The listing builds one solid part. Answer for the finished solid, in the listing's coordinates (mm). A direction names the side the tool comes from. Coordinates: 2 decimals unless noted, no trailing zeros. Order: outer loops, then holes, each group sorted by start corner. A loop starts at its lowest first (then second) coordinate and runs counter-clockwise, first axis right, second up. Notation, with made-up numbers: (-8.5, 15) -> (15.5, 15) arc R23 cw to (15.5, 23) -> close; hole circle Ø3 at (70, -28). An arc over 180 degrees is marked (long way). Return JSON: item names as keys, results as strings.
```python
from build123d import *

# Parameters (mm, degrees)
SKETCH2_R               = 6.1
BOSS_EXTRUDE1_DEPTH     = 30
SKETCH3_W               = 20
SKETCH3_H               = 20
BOSS_EXTRUDE2_DEPTH     = 5
SKETCH4_R               = 2.125
BOSS_EXTRUDE3_DEPTH     = 20
CUT_EXTRUDE1_DEPTH      = 20
CUT_EXTRUDE1_DEPTH_BACK = 20
SKETCH5_W               = 12.2
SKETCH5_H               = 16
FILLET2_R               = 10


with BuildPart() as part:
    # Sketch2 → Boss-Extrude1 (new body)
    with BuildSketch(Plane.XY):
        Circle(SKETCH2_R)
    extrude(amount=BOSS_EXTRUDE1_DEPTH)

    # Sketch3 → Boss-Extrude2 (add)
    with BuildSketch(Plane(origin=(0, 0, 0), x_dir=(-1, 0, 0), z_dir=(0, 0, -1))):
        Rectangle(SKETCH3_W, SKETCH3_H)
    extrude(amount=BOSS_EXTRUDE2_DEPTH)

    # Sketch4 → Boss-Extrude3 (add)
    with BuildSketch(Plane(origin=(10, 0, 0), x_dir=(0, 0, -1), z_dir=(1, 0, 0))):
        with BuildLine():
            Line((5, 0), (5, 5))
            Line((5, 5), (8, 5))
            ThreePointArc((8, 5), (13, 0), (8, -5))
            Line((8, -5), (5, -5))
            Line((5, -5), (5, 0))
        make_face()
        with Locations((8, 0)):
            Circle(SKETCH4_R, mode=Mode.SUBTRACT)
    extrude(amount=-BOSS_EXTRUDE3_DEPTH)

    # Sketch5 → Cut-Extrude1 (cut, two sides: drawn at the far end of the back side and taken through both)
    with BuildSketch(Plane(origin=(0, 0, 0), x_dir=(1, 0, 0), z_dir=(0, 1, 0)).offset(-CUT_EXTRUDE1_DEPTH_BACK)):
        with Locations((0, 13)):
            Rectangle(SKETCH5_W, SKETCH5_H)
    extrude(amount=CUT_EXTRUDE1_DEPTH + CUT_EXTRUDE1_DEPTH_BACK, mode=Mode.SUBTRACT)

    # Fillet2
    # the kernel refuses this fillet: 10 mm, written as the material it adds along each edge
    with BuildSketch(Plane(origin=(6.728171707, 5, -5), x_dir=(0, -0.09101222312672333, -0.9958497754388116), z_dir=(-1, 0, 0))) as fillet2_piece_1_section:
        with BuildLine():
            CenterArc((8.508585165, -9.412424416), FILLET2_R, 109.738733942, 43.945519562)
            Line((-0.455061116, -4.979248877), (-1.351425744, -4.535931323))
            ThreePointArc((-1.351425744, -4.535931323), (-1.223380333, -2.398612215), (-0.995849775, 0.091012223))
            Line((-0.995849775, 0.091012223), (0.091012223, 0.995849775))
            ThreePointArc((0.091012223, 0.995849775), (3.078561549, 0.722813106), (4.793537035, 0.941242442))
            Line((4.793537035, 0.941242442), (5.131268683, 0))
        make_face()
    fillet2_piece_1 = extrude(amount=16.728171707, mode=Mode.PRIVATE)
    fillet2_piece_1 = split(fillet2_piece_1, bisect_by=Plane(origin=(6.1, 6.116270273, -6.110221206), z_dir=(1, 0, 0)), keep=Keep.TOP, mode=Mode.PRIVATE)
    add(fillet2_piece_1)
    with BuildSketch(Plane(origin=(-6.1, 5, -5), x_dir=(0, -0.09101222312672332, -0.9958497754388116), z_dir=(-1, 0, 0))) as fillet2_piece_2:
        with BuildLine():
            CenterArc((8.508585165, -9.412424416), FILLET2_R, 109.738733942, 43.945519562)
            Line((-0.455061116, -4.979248877), (-1.351425744, -4.535931323))
            ThreePointArc((-1.351425744, -4.535931323), (-1.223380333, -2.398612215), (-0.995849775, 0.091012223))
            Line((-0.995849775, 0.091012223), (0.091012223, 0.995849775))
            ThreePointArc((0.091012223, 0.995849775), (3.078561549, 0.722813106), (4.793537035, 0.941242442))
            Line((4.793537035, 0.941242442), (5.131268683, 0))
        make_face()
    extrude(amount=3.9)
    with BuildSketch(Plane(origin=(10, 5, -5), x_dir=(0, 1, 0), z_dir=(-1, 0, 0))) as fillet2_piece_3:
        with BuildLine():
            CenterArc((8.598975489, 9.329918297), FILLET2_R, 204.960576151, 43.945519562)
            Line((-0.46700817, 5.109972766), (-1.373606536, 4.687978213))
            ThreePointArc((-1.373606536, 4.687978213), (-1, 3), (-1, 0))
            Line((-1, 0), (0, -1))
            ThreePointArc((0, -1), (2.5, -1), (4.640102451, -0.93299183))
            Line((4.640102451, -0.93299183), (5, 0))
        make_face()
    extrude(amount=3.9)
    with BuildSketch(Plane(origin=(10, 5, -5), x_dir=(0, 1, 0), z_dir=(-1, 0, 0))) as fillet2_piece_4_section:
        with BuildLine():
            CenterArc((8.598975489, 9.329918297), FILLET2_R, 204.960576151, 43.945519562)
            Line((-0.46700817, 5.109972766), (-1.373606536, 4.687978213))
            ThreePointArc((-1.373606536, 4.687978213), (-1, 3), (-1, 0))
            Line((-1, 0), (0, -1))
            ThreePointArc((0, -1), (2.5, -1), (4.640102451, -0.93299183))
            Line((4.640102451, -0.93299183), (5, 0))
        make_face()
    fillet2_piece_4 = extrude(amount=16.728171707, mode=Mode.PRIVATE)
    fillet2_piece_4 = split(fillet2_piece_4, bisect_by=Plane(origin=(-6.1, 6.116270273, -6.110221206), z_dir=(-1, 0, 0)), keep=Keep.TOP, mode=Mode.PRIVATE)
    add(fillet2_piece_4)
    with BuildSketch(Plane(origin=(6.728171707, -5, -5), x_dir=(0, 0.0910122231267235, -0.9958497754388116), z_dir=(-1, 0, 0))) as fillet2_piece_5_section:
        with BuildLine():
            CenterArc((8.508585165, 9.412424416), FILLET2_R, 206.315746496, 43.945519562)
            Line((-0.455061116, 4.979248877), (-1.351425744, 4.535931323))
            ThreePointArc((-1.351425744, 4.535931323), (-1.223380333, 2.398612215), (-0.995849775, -0.091012223))
            Line((-0.995849775, -0.091012223), (0.091012223, -0.995849775))
            ThreePointArc((0.091012223, -0.995849775), (3.078561549, -0.722813106), (4.793537035, -0.941242442))
            Line((4.793537035, -0.941242442), (5.131268683, 0))
        make_face()
    fillet2_piece_5 = extrude(amount=16.728171707, mode=Mode.PRIVATE)
    fillet2_piece_5 = split(fillet2_piece_5, bisect_by=Plane(origin=(6.1, -6.116270273, -6.110221206), z_dir=(1, 0, 0)), keep=Keep.TOP, mode=Mode.PRIVATE)
    add(fillet2_piece_5)
    with BuildSketch(Plane(origin=(-6.1, -5, -5), x_dir=(0, 0.0910122231267235, -0.9958497754388116), z_dir=(-1, 0, 0))) as fillet2_piece_6:
        with BuildLine():
            CenterArc((8.508585165, 9.412424416), FILLET2_R, 206.315746496, 43.945519562)
            Line((-0.455061116, 4.979248877), (-1.351425744, 4.535931323))
            ThreePointArc((-1.351425744, 4.535931323), (-1.223380333, 2.398612215), (-0.995849775, -0.091012223))
            Line((-0.995849775, -0.091012223), (0.091012223, -0.995849775))
            ThreePointArc((0.091012223, -0.995849775), (3.078561549, -0.722813106), (4.793537035, -0.941242442))
            Line((4.793537035, -0.941242442), (5.131268683, 0))
        make_face()
    extrude(amount=3.9)
    with BuildSketch(Plane(origin=(10, -5, -5), x_dir=(0, -1, 0), z_dir=(-1, 0, 0))) as fillet2_piece_7:
        with BuildLine():
            CenterArc((8.598975489, -9.329918297), FILLET2_R, 111.093904287, 43.945519562)
            Line((-0.46700817, -5.109972766), (-1.373606536, -4.687978213))
            ThreePointArc((-1.373606536, -4.687978213), (-1, -3), (-1, 0))
            Line((-1, 0), (0, 1))
            ThreePointArc((0, 1), (2.5, 1), (4.640102451, 0.93299183))
            Line((4.640102451, 0.93299183), (5, 0))
        make_face()
    extrude(amount=3.9)
    with BuildSketch(Plane(origin=(10, -5, -5), x_dir=(0, -1, 0), z_dir=(-1, 0, 0))) as fillet2_piece_8_section:
        with BuildLine():
            CenterArc((8.598975489, -9.329918297), FILLET2_R, 111.093904287, 43.945519562)
            Line((-0.46700817, -5.109972766), (-1.373606536, -4.687978213))
            ThreePointArc((-1.373606536, -4.687978213), (-1, -3), (-1, 0))
            Line((-1, 0), (0, 1))
            ThreePointArc((0, 1), (2.5, 1), (4.640102451, 0.93299183))
            Line((4.640102451, 0.93299183), (5, 0))
        make_face()
    fillet2_piece_8 = extrude(amount=16.728171707, mode=Mode.PRIVATE)
    fillet2_piece_8 = split(fillet2_piece_8, bisect_by=Plane(origin=(-6.1, -6.116270273, -6.110221206), z_dir=(-1, 0, 0)), keep=Keep.TOP, mode=Mode.PRIVATE)
    add(fillet2_piece_8)


solid = part.part
```
Item 1: Determine the mould class of faces 4 (the cylindrical face through (-8, 0, -13)), 5 (the flat face through (0, 10, -2)), 6 (the cylindrical face through (8.077, 1.792, -9.142)) for opening direction Y: pulls with the +Y half, pulls with the -Y half, needs draft (parallel to the pull), parting line crosses it, or undercut.
Answer list:
{"face 4": "parting line crosses it", "face 5": "pulls with the +Y half", "face 6": "undercut"}
Item 2: Which of the six approach directions +Z, -Z, +X, -X, +Y, -Y give full straight-line access (tool end or side, diameter ignored) to faces 1 (the cylindrical face through (-6.094, 0.268, 14.79)), 2 (the flat face through (-10, 0, -5)), 3 (the flat face through (0, 0, -5))?
Answer list:
{"face 1": "+Z", "face 2": "+Z, -Z, -X, +Y, -Y", "face 3": "-Z, +Y, -Y"}
Item 3: The part is cut by section A-A on y = 0. Determine the outline of the cut face in (x, z) (3 decimals), plus the area to 3 significant figures.
Answer list:
{"outline": "(-10, -13) -> (-6.1, -13) -> (-6.1, -10.125) -> (-10, -10.125) -> close; (-10, -5.875) -> (-6.1, -5.875) -> (-6.1, -5) -> (6.1, -5) -> (6.1, -5.875) -> (10, -5.875) -> (10, 0) -> (6.1, 0) -> (6.1, 30) -> (-6.1, 30) -> (-6.1, 0) -> (-10, 0) -> close; (6.1, -13) -> (10, -13) -> (10, -10.125) -> (6.1, -10.125) -> close", "area": "495 mm2"}
Item 4: The part is cut by section B-B on x = 8.5. Determine the outline of the cut face in (y, z) (3 decimals), plus the area to 3 significant figures.
Answer list:
{"outline": "(-10, -5) arc R10 cw to (-4.533, -10.11) arc R5 ccw to (4.533, -10.11) arc R10 cw to (10, -5) -> (10, 0) -> (-10, 0) -> close; hole circle Ø4.25 at (0, -8)", "area": "172 mm2"}
Item 5: The part is cut by section C-C on z = -8. Determine the outline of the cut face in (x, y) (3 decimals).
Answer list:
{"outline": "(-10, -5.857) -> (-6.1, -5.857) -> (-6.1, -2.125) -> (-10, -2.125) -> close; (-10, 2.125) -> (-6.1, 2.125) -> (-6.1, 5.857) -> (-10, 5.857) -> close; (6.1, -5.857) -> (10, -5.857) -> (10, -2.125) -> (6.1, -2.125) -> close; (6.1, 2.125) -> (10, 2.125) -> (10, 5.857) -> (6.1, 5.857) -> close"}
Item 6: Find the intervals of material crossed by probe 1 along Z at (x, y) = (0, -2); probe 2 along Z at (x, y) = (-1.5, -8); probe 3 along X at (y, z) = (2, -11), in increasing order.
Answer list:
{"probe 1": "-5 to 30", "probe 2": "-5 to 0", "probe 3": "-10 to -6.1, 6.1 to 10"}
Item 7: Flat-ended cylindrical pins translate along their axes: pin 1 (10 mm diameter, centred on x = -8, y = 8, fed in from +Z); pin 2 (10 mm diameter, centred on x = 1, z = 21.5, fed in from -Y); pin 3 (1 mm diameter, centred on y = 0.5, z = 5, fed in from +X). Find the tip coordinate at first contact, or state that the pin passes through.
Answer list:
{"pin 1": "z = 0", "pin 2": "y = -6.1", "pin 3": "x = 6.1"}
Item 8: The part is cut by section D-D on x = 3.5. Determine the outline of the cut face in (y, z).
Answer list:
{"outline": "(-10, -5) -> (10, -5) -> (10, 0) -> (5, 0) -> (5, 30) -> (-5, 30) -> (-5, 0) -> (-10, 0) -> close"}
